Input: dimensioned drawing with shaded views. Units: mm. Origin: part minimum x, y, z. A direction names the side the tool comes from. Coordinates: 2 decimals unless noted, no trailing zeros. Write each loop counter-clockwise with the first axis right and the second up, starting at its lowest first coordinate (ties: lowest second). Pieces come first, ordered by that corner, then holes. Notation, with made-up numbers: M 43.25,-18 L 84.25,-18 A19 ccw 84.25,-14 Z; hole C -35,77.25 d3. An arc over 180 degrees is marked long. Use one line per item in the form item = value.
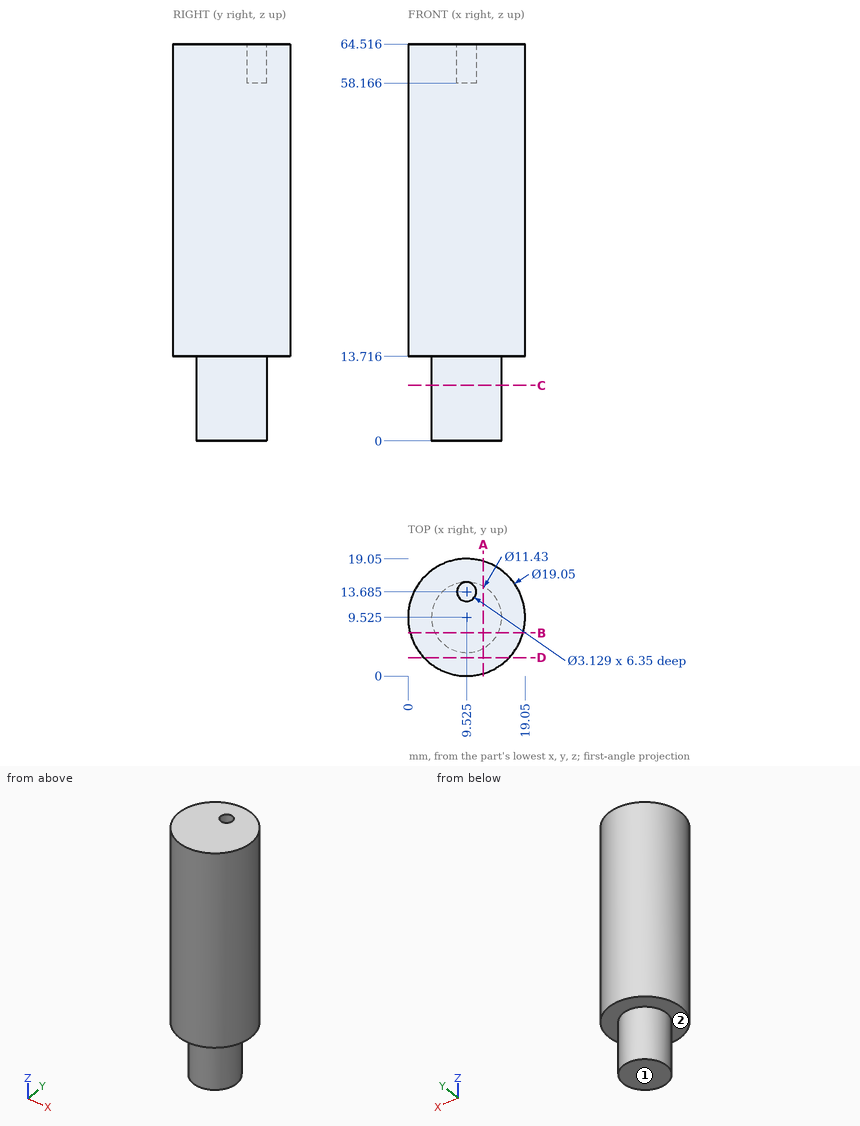
(1) Line query: probe 1 along Z at (x, y) = (17, 4.75); probe 2 along X at (y, z) = (14, 58.5) (1 decimal); probe 3 along X at (y, z) = (10, 49). Output: solid intervals per line, ascending.
Computed:
probe_1 = 13.72 to 64.52
probe_2 = 1.1 to 8, 11.1 to 17.9
probe_3 = 0.01 to 19.04
(2) Section query D-D on y = 3. Return the cut outline in (x, z).
Computed:
outline = M 2.59,13.72 L 16.46,13.72 L 16.46,64.52 L 2.59,64.52 Z
(3) Section query A-A on x = 12.25. Return the cut outline in (y, z), plus the area to 4 significant figures.
Computed:
outline = M 0.4,13.72 L 4.5,13.72 L 4.5,0 L 14.55,0 L 14.55,13.72 L 18.65,13.72 L 18.65,64.52 L 0.4,64.52 Z
area = 1,065 mm^2
(4) Set-up query: the marked faces 1 and 2. Return all of +Z, -Z, +X, -X, +Y, -Y with unobstructed straight access to the full face (end or side cutting, diameter ignored); none if empty.
Computed:
face_1 = -Z, +X, -X, +Y, -Y
face_2 = -Z
(5) Section query B-B on y = 7. Return the cut outline in (x, z).
Computed:
outline = M 0.34,13.72 L 4.4,13.72 L 4.4,0 L 14.65,0 L 14.65,13.72 L 18.71,13.72 L 18.71,64.52 L 0.34,64.52 Z
(6) Section query C-C on z = 9. Return the cut outline in (x, y) (1 decimal), plus the area to 3 significant figures.
Computed:
outline = C 9.5,9.5 d11.4
area = 103 mm^2
(7) First-contact query: pin 1 Ø1.5 at (x, z) = (8, 44.5) entering from +Y; pin 2 Ø1.6 at (x, y) = (10, 14) entering from +Z; pin 3 Ø5 at (x, z) = (16, 52) entering from -Y. Flat tips, straight axial feed; report the tip coordinate or a pass-through.
Computed:
pin_1 = 19.02
pin_2 = 58.17
pin_3 = 0.87
